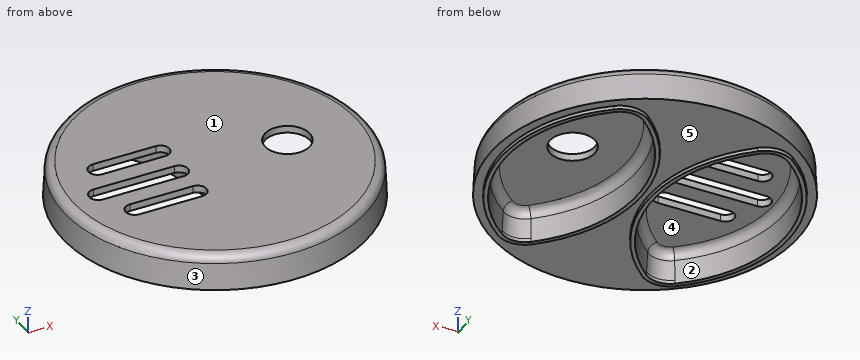
```python
from build123d import *

# Parameters (mm, degrees)
F0_R      = 34
F1_DEPTH  = 8
F1_TAPER  = 3
F3_DEPTH  = 6.4
F3_TAPER  = 3
F5_DEPTH  = 0.8
F5_TAPER  = 3
F6_R      = 2
F8_D      = 10
F10_DEPTH = 8.8010001
F12_DEPTH = 8.8010001


with BuildPart() as f1:
    # F0 (on Top) → F1 (new body)
    with BuildSketch(Plane.XY):
        Circle(F0_R)
    extrude(amount=F1_DEPTH, taper=F1_TAPER)

    # F2 (on face) → F3 (cut)
    with BuildSketch(Plane(origin=(0, 0, 0), x_dir=(1, 0, 0), z_dir=(0, 0, -1))):
        with BuildLine():
            ThreePointArc((-12.8411571335, 24.1811270559), (-16.0020129755, 25.4015270201), (-19.2152025489, 24.3264463291))
            ThreePointArc((-19.2152025489, 24.3264463291), (-31, 0), (-19.2152025489, -24.3264463291))
            ThreePointArc((-19.2152025489, -24.3264463291), (-16.0020129755, -25.4015270201), (-12.8411571335, -24.1811270559))
            ThreePointArc((-12.8411571335, -24.1811270559), (-1.8, 0), (-12.8411571335, 24.1811270559))
        make_face()
        with BuildLine():
            ThreePointArc((12.8411571335, 24.1811270559), (1.8, 0), (12.8411571335, -24.1811270559))
            ThreePointArc((12.8411571335, -24.1811270559), (16.0020129755, -25.4015270201), (19.2152025489, -24.3264463291))
            ThreePointArc((19.2152025489, -24.3264463291), (31, 0), (19.2152025489, 24.3264463291))
            ThreePointArc((19.2152025489, 24.3264463291), (16.0020129755, 25.4015270201), (12.8411571335, 24.1811270559))
        make_face()
    extrude(amount=-F3_DEPTH, taper=F3_TAPER, mode=Mode.SUBTRACT)

    # F4 (on face) → F5 (join)
    with BuildSketch(Plane(origin=(0, 0, 0), x_dir=(1, 0, 0), z_dir=(0, 0, -1))):
        with BuildLine():
            ThreePointArc((-12.1861932939, -24.9367872764), (-0.8, 0), (-12.1861932939, 24.9367872764))
            ThreePointArc((-12.1861932939, 24.9367872764), (-15.9792203044, 26.4012672334), (-19.8350477924, 25.1111704043))
            ThreePointArc((-19.8350477924, 25.1111704043), (-32, 0), (-19.8350477924, -25.1111704043))
            ThreePointArc((-19.8350477924, -25.1111704043), (-15.9792203044, -26.4012672334), (-12.1861932939, -24.9367872764))
        make_face()
        with BuildLine():
            ThreePointArc((-19.2152025489, -24.3264463291), (-31, 0), (-19.2152025489, 24.3264463291))
            ThreePointArc((-19.2152025489, 24.3264463291), (-16.0020129755, 25.4015270201), (-12.8411571335, 24.1811270559))
            ThreePointArc((-12.8411571335, 24.1811270559), (-1.8, 0), (-12.8411571335, -24.1811270559))
            ThreePointArc((-12.8411571335, -24.1811270559), (-16.0020129755, -25.4015270201), (-19.2152025489, -24.3264463291))
        make_face(mode=Mode.SUBTRACT)
        with BuildLine():
            ThreePointArc((19.8350477924, -25.1111704043), (32, 0), (19.8350477924, 25.1111704043))
            ThreePointArc((19.8350477924, 25.1111704043), (15.9792203044, 26.4012672334), (12.1861932939, 24.9367872764))
            ThreePointArc((12.1861932939, 24.9367872764), (0.8, 0), (12.1861932939, -24.9367872764))
            ThreePointArc((12.1861932939, -24.9367872764), (15.9792203044, -26.4012672334), (19.8350477924, -25.1111704043))
        make_face()
        with BuildLine():
            ThreePointArc((12.8411571335, 24.1811270559), (16.0020129755, 25.4015270201), (19.2152025489, 24.3264463291))
            ThreePointArc((19.2152025489, 24.3264463291), (31, 0), (19.2152025489, -24.3264463291))
            ThreePointArc((19.2152025489, -24.3264463291), (16.0020129755, -25.4015270201), (12.8411571335, -24.1811270559))
            ThreePointArc((12.8411571335, -24.1811270559), (1.8, 0), (12.8411571335, 24.1811270559))
        make_face(mode=Mode.SUBTRACT)
    extrude(amount=F5_DEPTH, taper=F5_TAPER)

    # F6
    f6_edges = [f1.edges().sort_by_distance(p)[0] for p in [
        (-33.580738, 0, 8),
        (-30.66459, 0, 6.4),
        (2.13541, 0, 6.4),
    ]]
    fillet(f6_edges, radius=F6_R)

    # F8 (through all)
    with Locations(Plane.XY.offset(8)):
        with Locations((16.1159763314, 0)):
            Hole(F8_D / 2)

    # F9 (on face) → F10 (cut, through all)
    with BuildSketch(Plane.XY.offset(8)):
        with BuildLine():
            Line((-26, -2), (-8, -2))
            ThreePointArc((-8, -2), (-6, 0), (-8, 2))
            Line((-8, 2), (-26, 2))
            ThreePointArc((-26, 2), (-28, 0), (-26, -2))
        make_face()
    extrude(amount=-F10_DEPTH, mode=Mode.SUBTRACT)

    # F11 (on face) → F12 (cut, through all)
    with BuildSketch(Plane.XY.offset(8)):
        with BuildLine():
            Line((-22, 6), (-8, 6))
            ThreePointArc((-8, 6), (-6, 8), (-8, 10))
            Line((-8, 10), (-22, 10))
            ThreePointArc((-22, 10), (-24, 8), (-22, 6))
        make_face()
        with BuildLine():
            ThreePointArc((-8, -10), (-6, -8), (-8, -6))
            Line((-8, -6), (-22, -6))
            ThreePointArc((-22, -6), (-24, -8), (-22, -10))
            Line((-22, -10), (-8, -10))
        make_face()
    extrude(amount=-F12_DEPTH, mode=Mode.SUBTRACT)


solid = f1.part
```
Here's how the part is built. I have some questions about the finished solid (model axes, mm). Face numbers are marked on the shaded views. A direction names the side the tool comes from. Round coordinates to 2 decimals unless told otherwise and drop trailing zeros. Answer as CSV lines item,"result". Start each with the question number.
1. I'm going to push flat-ended pins straight in: pin 1 Ø0.5 at (x, z) = (-21.5, 7.5) entering from +Y; pin 2 Ø1.5 at (y, z) = (6.5, 0) entering from +X; pin 3 Ø1.3 at (x, z) = (-14.5, 7.5) entering from -Y. Where does each tip first touch, or does it pass through?
2. I need wall thicknesses on probe 1 along X at (y, z) = (-20, 2.5); probe 2 along X at (y, z) = (-12.5, 4.25); probe 3 along Z at (x, y) = (-6, 28.5). Which ranges of each line are inside material? Lowest first, please.
3. Thinking about a two-plate mould opening in Y: for the marked faces 3, 4 and 5, which applies, released by +Y, released by -Y, zero draft, split by the parting line, or undercut?
4. Suppose I cut it at A-A on y = 0. Count the separate pieces of the cut face and the enclosed holes in it, then the cut area to 3 significant figures.
5. On a 3-axis mill with a long thin cutter (end or side, diameter ignored), from which of +Z, -Z, +X, -X, +Y, -Y can I reach the whole of each face in a straight line? I mean the marked faces 1 and 2. Say none if no direction works.
Check result:
1,pin 1,"stops at y = 25.43"
1,pin 2,"stops at x = 33.51"
1,pin 3,"stops at y = -30.3"
2,probe 1,"x = -27.33 to -23.51, -8.99 to 8.99, 23.51 to 27.33"
2,probe 2,"x = -31.38 to -28.12, -4.58 to 4.58, 28.12 to 31.38"
2,probe 3,"z = 0 to 8"
3,face 3,"split by the parting line"
3,face 4,"undercut"
3,face 5,"zero draft"
4,separate pieces,"3"
4,enclosed holes,"0"
4,area,"125 mm2"
5,face 1,"+Z, +X, -X, +Y, -Y"
5,face 2,"-Z"
